from build123d import *

# Parameters (mm, degrees)
F1_DEPTH     = 8
F0_W         = 14.25
F0_H         = 4
F0_W_2       = 5
F2_DEPTH     = 0.4
F3_T1_DEPTH  = 6
F3_T8_ANGLE  = 180
F3_T10_ANGLE = 180
F3_T12_ANGLE = 180
F3_T14_ANGLE = 180
F4_R         = 4.5
F4_W         = 8.75
F4_H         = 8.75
F5_DEPTH     = 4
F6_F1_R      = 1
F6_F2_R      = 1


# Not quite as in the source:
# - a fillet or chamfer that OpenCascade refuses, or shapes differently, is made with other operations: its cross-section is extruded or revolved along the edge and cut away or added


with BuildPart() as f1:
    # F0 (on Top) → F1 (new body)
    with BuildSketch(Plane.XY):
        Polygon((13.25, 2), (13.25, 13.25), (-13.25, 13.25), (-13.25, -13.25), (13.25, -13.25), (13.25, -2), align=None)
    extrude(amount=F1_DEPTH)



with BuildPart() as f1b:
    # F0 (on Top) → F1, piece 2 (new body)
    with BuildSketch(Plane.XY):
        with BuildLine():
            ThreePointArc((76.9282032303, 12), (70.3656241563, 16.7495627838), (67.9048645752, 9.0313730334))
            ThreePointArc((67.9048645752, 9.0313730334), (69.4282032303, 7.6698729811), (71.3689661904, 7.0313730334))
            ThreePointArc((71.3689661904, 7.0313730334), (75.260155721, 8.2719854346), (76.9282032303, 12))
        make_face()
    extrude(amount=F1_DEPTH)


with BuildPart() as f1c:
    # F0 (on Top) → F1, piece 3 (new body)
    with BuildSketch(Plane.XY):
        with BuildLine():
            ThreePointArc((62.0951354248, -9.0313730334), (60.5717967697, -7.6698729811), (58.6310338096, -7.0313730334))
            ThreePointArc((58.6310338096, -7.0313730334), (54.3437822043, -15.3319524907), (63.0717967697, -12))
            ThreePointArc((63.0717967697, -12), (62.8213595536, -10.437420926), (62.0951354248, -9.0313730334))
        make_face()
    extrude(amount=F1_DEPTH)


with BuildPart() as f1d:
    # F0 (on Top) → F1, piece 4 (new body)
    with BuildSketch(Plane.XY):
        with BuildLine():
            Line((27.5, 3), (27.5, 2))
            Line((27.5, 2), (27.5, -2))
            Line((27.5, -2), (27.5, -3))
            ThreePointArc((27.5, -3), (30, -5.5), (32.5, -3))
            Line((32.5, -3), (32.5, -2))
            Line((32.5, -2), (32.5, 2))
            Line((32.5, 2), (32.5, 3))
            ThreePointArc((32.5, 3), (30, 5.5), (27.5, 3))
        make_face()
    extrude(amount=F1_DEPTH)


with BuildPart() as f1e:
    # F0 (on Top) → F1, piece 5 (new body)
    with BuildSketch(Plane.XY):
        with BuildLine():
            Line((37.5, 3), (37.5, 2))
            Line((37.5, 2), (37.5, -2))
            Line((37.5, -2), (37.5, -3))
            ThreePointArc((37.5, -3), (40, -5.5), (42.5, -3))
            Line((42.5, -3), (42.5, -2))
            Line((42.5, -2), (42.5, 2))
            Line((42.5, 2), (42.5, 3))
            ThreePointArc((42.5, 3), (40, 5.5), (37.5, 3))
        make_face()
    extrude(amount=F1_DEPTH)


with BuildPart() as f1_1:
    add(f1.part)

    add(f1b.part)  # F2 merges F1b

    add(f1c.part)  # F2 merges F1c

    add(f1d.part)  # F2 merges F1d

    add(f1e.part)  # F2 merges F1e
    # F0 (on Top) → F2 (join)
    with BuildSketch(Plane.XY):
        with Locations((20.375, 0)):
            Rectangle(F0_W, F0_H)
        with Locations((35, 0)):
            Rectangle(F0_W_2, F0_H)
        Polygon((63.8452994616, 2), (42.5, 2), (42.5, -2), (61.5358983849, -2), align=None)
        with BuildLine():
            Line((67.9048645752, 9.0313730334), (63.8452994616, 2))
            Line((63.8452994616, 2), (61.5358983849, -2))
            Line((61.5358983849, -2), (58.6310338096, -7.0313730334))
            ThreePointArc((58.6310338096, -7.0313730334), (60.5717967697, -7.6698729811), (62.0951354248, -9.0313730334))
            Line((62.0951354248, -9.0313730334), (71.3689661904, 7.0313730334))
            ThreePointArc((71.3689661904, 7.0313730334), (69.4282032303, 7.6698729811), (67.9048645752, 9.0313730334))
        make_face()
    extrude(amount=F2_DEPTH)

    # F3: fillet of radius 2.5 on 10 edges, made by hand

    # F3_s2 → F3_t1 (cut)
    with BuildSketch(Plane.XZ.offset(-3)):
        with BuildLine():
            ThreePointArc((37.5, 5.5), (38.232233047, 7.267766953), (40, 8))
            Line((40, 8), (37.5, 8))
            Line((37.5, 8), (37.5, 5.5))
        make_face()
        with BuildLine():
            ThreePointArc((42.5, 5.5), (41.767766953, 7.267766953), (40, 8))
            Line((40, 8), (42.5, 8))
            Line((42.5, 8), (42.5, 5.5))
        make_face()
        with BuildLine():
            ThreePointArc((27.5, 5.5), (28.232233047, 7.267766953), (30, 8))
            Line((30, 8), (27.5, 8))
            Line((27.5, 8), (27.5, 5.5))
        make_face()
        with BuildLine():
            ThreePointArc((32.5, 5.5), (31.767766953, 7.267766953), (30, 8))
            Line((30, 8), (32.5, 8))
            Line((32.5, 8), (32.5, 5.5))
        make_face()
    extrude(amount=F3_T1_DEPTH, mode=Mode.SUBTRACT)

    # F3_s3 → F3_t4 (revolve, cut)
    with BuildSketch(Plane.XZ.offset(12)):
        with BuildLine():
            ThreePointArc((63.0717967697, 5.5), (62.3395637227, 7.267766953), (60.5717967697, 8))
            Line((60.5717967697, 8), (63.0717967697, 8))
            Line((63.0717967697, 8), (63.0717967697, 5.5))
        make_face()
    revolve(axis=Axis((58.0717967697, -12, 8), (0, 0, -1)), mode=Mode.SUBTRACT)

    # F3_s5 → F3_t6 (revolve, cut)
    with BuildSketch(Plane(origin=(19.6223796234, -26.5939369719, 0), x_dir=(0, 0, 1), z_dir=(0.5937253933, -0.804667731, 0))):
        with BuildLine():
            ThreePointArc((5.5, -60.0030088087), (7.267766953, -60.7352418558), (8, -62.5030088087))
            Line((8, -62.5030088087), (8, -60.0030088087))
            Line((8, -60.0030088087), (5.5, -60.0030088087))
        make_face()
    revolve(axis=Axis((71.9282032303, 12, 8), (0, 0, -1)), mode=Mode.SUBTRACT)

    # F3_s7 → F3_t8 (revolve, cut)
    with BuildSketch(Plane.XZ.offset(-3)):
        with BuildLine():
            ThreePointArc((42.5, 5.5), (41.767766953, 7.267766953), (40, 8))
            Line((40, 8), (42.5, 8))
            Line((42.5, 8), (42.5, 5.5))
        make_face()
    revolve(axis=Axis((40, 3, 8), (0, 0, 1)), revolution_arc=F3_T8_ANGLE, mode=Mode.SUBTRACT)

    # F3_s9 → F3_t10 (revolve, cut)
    with BuildSketch(Plane.XZ.offset(3)):
        with BuildLine():
            ThreePointArc((40, 8), (38.232233047, 7.267766953), (37.5, 5.5))
            Line((37.5, 5.5), (37.5, 8))
            Line((37.5, 8), (40, 8))
        make_face()
    revolve(axis=Axis((40, -3, 8), (0, 0, 1)), revolution_arc=F3_T10_ANGLE, mode=Mode.SUBTRACT)

    # F3_s11 → F3_t12 (revolve, cut)
    with BuildSketch(Plane.XZ.offset(-3)):
        with BuildLine():
            ThreePointArc((32.5, 5.5), (31.767766953, 7.267766953), (30, 8))
            Line((30, 8), (32.5, 8))
            Line((32.5, 8), (32.5, 5.5))
        make_face()
    revolve(axis=Axis((30, 3, 8), (0, 0, 1)), revolution_arc=F3_T12_ANGLE, mode=Mode.SUBTRACT)

    # F3_s13 → F3_t14 (revolve, cut)
    with BuildSketch(Plane.XZ.offset(3)):
        with BuildLine():
            ThreePointArc((27.5, 5.5), (28.232233047, 7.267766953), (30, 8))
            Line((30, 8), (27.5, 8))
            Line((27.5, 8), (27.5, 5.5))
        make_face()
    revolve(axis=Axis((30, -3, 8), (0, 0, 1)), revolution_arc=F3_T14_ANGLE, mode=Mode.SUBTRACT)

    # F4 (on face) → F5 (cut)
    with BuildSketch(Plane.XY.offset(8)):
        Circle(F4_R)
        with Locations((-8.875, 8.875)):
            Rectangle(F4_W, F4_H)
        with Locations((-8.875, -8.875)):
            Rectangle(F4_W, F4_H)
        with Locations((8.875, -8.875)):
            Rectangle(F4_W, F4_H)
        with Locations((8.875, 8.875)):
            Rectangle(F4_W, F4_H)
    extrude(amount=-F5_DEPTH, mode=Mode.SUBTRACT)

    # F6: fillet of radius 1 on 16 edges, made by hand

    # F6_f1
    f6_f1_edges = [f1_1.edges().sort_by_distance(p)[0] for p in [
        (8.875, -4.5, 4),
        (4.5, -8.875, 4),
        (4.5, 8.875, 4),
        (8.875, 4.5, 4),
        (-4.5, 8.875, 4),
        (-8.875, 4.5, 4),
        (-8.875, -4.5, 4),
        (-4.5, -8.875, 4),
    ]]
    fillet(f6_f1_edges, radius=F6_F1_R)

    # F6_f2
    f6_f2_edges = [f1_1.edges().sort_by_distance(p)[0] for p in [
        (13.25, -9.375, 4),
        (9.375, -13.25, 4),
        (9.375, 13.25, 4),
        (13.25, 9.375, 4),
        (-9.375, 13.25, 4),
        (-13.25, 9.375, 4),
        (-13.25, -9.375, 4),
        (-9.375, -13.25, 4),
        (-4.7928932188, -13.25, 4.2928932188),
        (-13.25, -4.7928932188, 4.2928932188),
        (-13.25, 4.7928932188, 4.2928932188),
        (-4.7928932188, 13.25, 4.2928932188),
        (13.25, 4.7928932188, 4.2928932188),
        (4.7928932188, 13.25, 4.2928932188),
        (4.7928932188, -13.25, 4.2928932188),
        (13.25, -4.7928932188, 4.2928932188),
    ]]
    fillet(f6_f2_edges, radius=F6_F2_R)


solid = f1_1.part
Design review of the part built by this model. Coordinates are the model's own, in mm. A direction names the side the tool comes from. Coordinates: 2 decimals unless noted, no trailing zeros. Loops run counter-clockwise (first coordinate to the right, second up) from the corner with the lowest first, then second, coordinate; pieces in that order, holes last. Notation, with made-up numbers: M -19.5,22 L 20.5,22 A15 ccw 20.5,45 Z; hole C 12.25,-12 d2. An arc over 180 degrees is marked long. Answer as CSV lines item,"result".
Item 1: For P1, Ø3.5, axis at y = 8.5, z = 6, coming from the -X side; P2, Ø10, axis at x = 2, y = 1.5, coming from the +Z side; P3, Ø3, axis at y = 10, z = 4.5, coming from the +X side; P4, Ø3, axis at x = 5.5, z = 4, coming from the +Y side, all flat-tipped, find the tip position at first contact; note any pin that passes through.
Answer list:
P1,"x = -4.84"
P2,"z = 8"
P3,"x = 76.9"
P4,"y = 13.25"
Item 2: Add section B-B on x = 0. State the section outline as (y, z) points, plus the area to 3 significant figures.
Answer list:
outline,"M -13.25,0 L 13.25,0 L 13.25,8 L 4.5,8 L 4.5,4 L -4.5,4 L -4.5,8 L -13.25,8 Z"
area,"176 mm²"
Item 3: Machinability: for faces 1 (the face through (-8, 4.5, 7)), 2 (the face through (8, -4.5, 7)), 3 (the face through (9, 9, 4)), 4 (the face through (-13.25, 0, 3)), which of the approach directions +Z, -Z, +X, -X, +Y, -Y give a long, thin tool a straight path to every point of the face, cutting with its end or side? Answer none if there is none.
Answer list:
face 1,"+Z, -X, +Y"
face 2,"+Z, -Y"
face 3,"+Z, +Y"
face 4,"+Z, -Z, -X, +Y, -Y"
Item 4: Add section C-C on y = 0. State the section outline as (x, z) points, plus the area to 3 significant figures.
Answer list:
outline,"M -13.25,0 L 67.31,0 L 67.31,0.4 L 42.5,0.4 L 42.5,5.5 A2.5 ccw 37.5,5.5 L 37.5,0.4 L 32.5,0.4 L 32.5,5.5 A2.5 ccw 27.5,5.5 L 27.5,0.4 L 13.25,0.4 L 13.25,8 L 4.5,8 L 4.5,4 L -4.5,4 L -4.5,8 L -13.25,8 Z"
area,"268 mm²"
Item 5: The part is to be moulded in two halves that separate along Y. For faces 5 (the face through (60.104, -4.48, 0.197)), 6 (the face through (-4.5, 8, 7)), 7 (the face through (0, -13.25, 3)), 8 (the face through (40.1, 5.5, 2.7)), say which applies: pulls with the +Y half, pulls with the -Y half, needs draft (parallel to the pull), parting line crosses it, or undercut.
Answer list:
face 5,"undercut"
face 6,"needs draft"
face 7,"pulls with the -Y half"
face 8,"pulls with the +Y half"
Item 6: For probe 1 along X at (y, z) = (-1, 6); probe 2 along Y at (x, z) = (0, 5.3); probe 3 along X at (y, z) = (7, 7.75), list the stretches that pass through material, from the lowest coordinate up.
Answer list:
probe 1,"-13.25 to -4.39, 4.39 to 13.25, 27.55 to 32.45, 37.55 to 42.45"
probe 2,"-13.25 to -4.5, 4.5 to 13.25"
probe 3,"-4.5 to 4.5"
Item 7: Add section D-D on z = 6.5. Count the separate pieces of the cut face and the enclosed holes in it, plus the area to 3 significant figures.
Answer list:
separate pieces,"5"
enclosed holes,"1"
area,"563 mm²"
Item 8: Add section A-A on z = 2. State the section outline as (x, y) points.
Answer list:
outline,"M -13.25,-13.25 L 13.25,-13.25 L 13.25,13.25 L -13.25,13.25 Z; M 27.5,-3 A2.5 ccw 32.5,-3 L 32.5,3 A2.5 ccw 27.5,3 Z; M 37.5,-3 A2.5 ccw 42.5,-3 L 42.5,3 A2.5 ccw 37.5,3 Z; C 58.07,-12 d10; C 71.93,12 d10"
